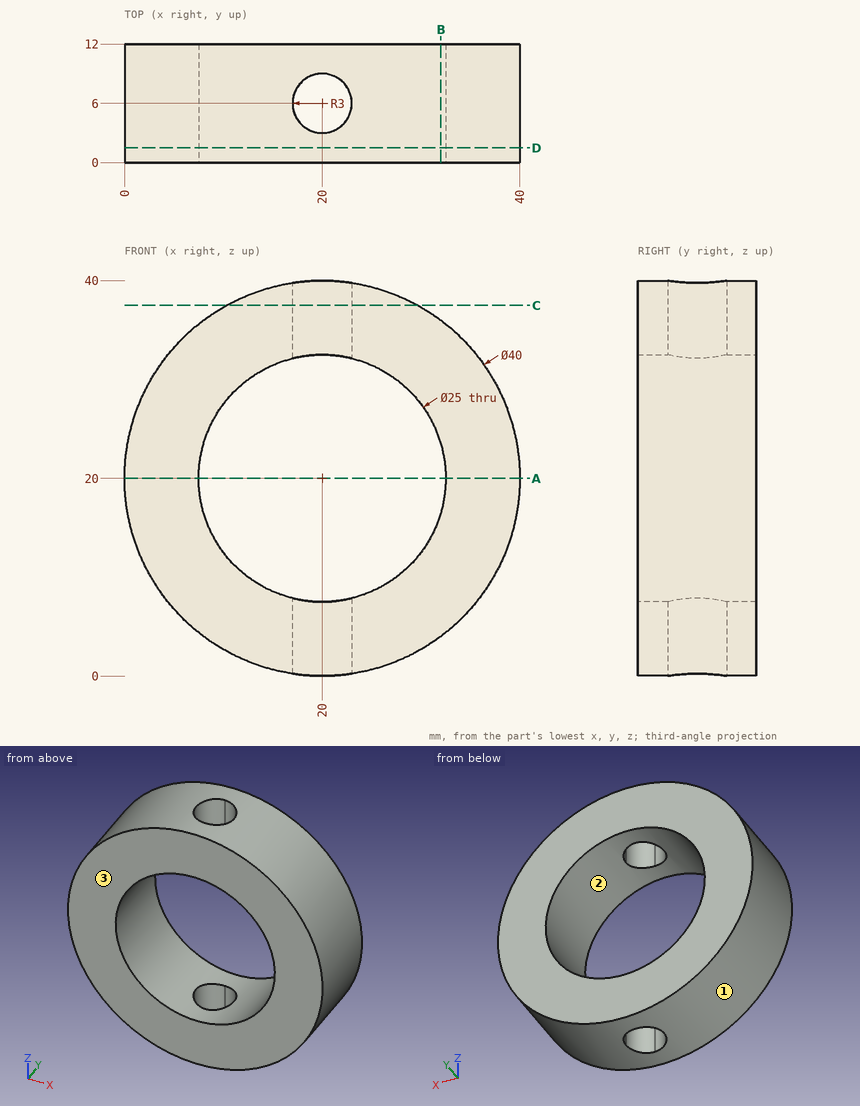
Verification items for this drawing (mm, ordinates from the low corner). Coordinates: 2 decimals unless noted, no trailing zeros. Write each loop counter-clockwise with the first axis right and the second up, starting at its lowest first coordinate (ties: lowest second). Pieces come first, ordered by that corner, then holes. Notation, with made-up numbers: (-32, 36) -> (-13, 36) arc R24 cw to (-13, 55) -> close; hole circle Ø3 at (74.25, 8.5). An arc over 180 degrees is marked (long way). One line per item, written item: value. Start each with the question number.
Q1. Mould release check, pull along X, two halves, no side actions. Record for the marked faces 1, 2 and 3: pulls with the +X half, pulls with the -X half, needs draft (parallel to the pull), parting line crosses it, or undercut.
Q2. Cross-section at A-A on z = 20. Enter the section's corners in (x, y).
Q3. Cross-section at B-B on x = 32. Enter the section's corners in (y, z), and give its area (3 significant figures).
Q4. Cross-section at D-D on y = 1.5. Enter the section's corners in (x, z), and give its area (3 significant figures).
Q5. Go/stop test with flat-tipped pins: P1, Ø1, axis at x = 19, y = 6.5, coming from the +Z side; P2, Ø6, axis at x = 12, y = 6.5, coming from the +Z side; P3, Ø3, axis at x = 5, y = 5.5, coming from the +Z side; P4, Ø3, axis at x = 26.5, z = 11, coming from the +Y side. Record where each tip stops, or that it passes through.
Q6. Cross-section at C-C on z = 37.5. Enter the section's corners in (x, y), and give its area (3 significant figures).
Q7. Thickness scan on L1, parallel to X at y = 9.75, z = 20; L2, parallel to Z at x = 26.5, y = 3.75; L3, parallel to Y at x = 18, z = 36. Record the ranges inside material, lowest first. Write a range as from..to.
Checked values:
1. face 1: parting line crosses it
1. face 2: undercut
1. face 3: needs draft
2. outline: (0, 0) -> (7.5, 0) -> (7.5, 12) -> (0, 12) -> close; (32.5, 0) -> (40, 0) -> (40, 12) -> (32.5, 12) -> close
3. outline: (0, 4) -> (12, 4) -> (12, 16.5) -> (0, 16.5) -> close; (0, 23.5) -> (12, 23.5) -> (12, 36) -> (0, 36) -> close
3. area: 300 mm²
4. outline: circle Ø40 at (20, 20); hole circle Ø25 at (20, 20)
4. area: 766 mm²
5. P1: passes through
5. P2: stops at z = 39.36
5. P3: stops at z = 34.76
5. P4: stops at y = 12
6. outline: (10.32, 0) -> (29.68, 0) -> (29.68, 12) -> (10.32, 12) -> close; hole circle Ø6 at (20, 6)
6. area: 204 mm²
7. L1: x = 0..7.5, 32.5..40
7. L2: z = 1.09..9.32, 30.68..38.91
7. L3: y = 0..3.76, 8.24..12
